```python
from build123d import *

# Parameters (mm, degrees)
F1_DEPTH = 24
F2_R     = 1.98374
F3_R     = 3.69316
F4_R     = 3.96875
F5_R     = 0.762
F6_R     = 1.8288
F7_DEPTH = 1.70942


with BuildPart() as f1:
    # F0 (on Top) → F1 (new body)
    with BuildSketch(Plane.XY):
        Polygon((0, -13.29058), (0, 0), (9.92124, 0), (9.92124, 1.70942), (-1.70942, 1.70942), (-1.70942, -11.58116), (-16.70942, -11.58116), (-16.70942, -13.29058), align=None)
    extrude(amount=F1_DEPTH)

    # F2
    f2_edges = [f1.edges().sort_by_distance(p)[0] for p in [
        (0, 0, 12),
        (-1.70942, -11.58116, 12),
    ]]
    fillet(f2_edges, radius=F2_R)

    # F3
    f3_edges = [f1.edges().sort_by_distance(p)[0] for p in [
        (0, -13.29058, 12),
        (-1.70942, 1.70942, 12),
    ]]
    fillet(f3_edges, radius=F3_R)

    # F4
    f4_edges = [f1.edges().sort_by_distance(p)[0] for p in [
        (9.92124, 0.85471, 24),
        (9.92124, 0.85471, 0),
    ]]
    fillet(f4_edges, radius=F4_R)

    # F5
    f5_edges = [f1.edges().sort_by_distance(p)[0] for p in [
        (-16.70942, -12.43587, 0),
        (-16.70942, -12.43587, 24),
    ]]
    fillet(f5_edges, radius=F5_R)

    # F6 (on face) → F7 (cut, through all)
    with BuildSketch(Plane.XZ):
        with Locations((5.95249, 20.03125)):
            Circle(F6_R)
        with Locations((5.95249, 3.96875)):
            Circle(F6_R)
    extrude(amount=-F7_DEPTH, mode=Mode.SUBTRACT)


solid = f1.part
```
The model under review builds one solid part; all positions refer to its coordinate system, in mm. A direction names the side the tool comes from. Give positions to 0.01 mm unless a question says otherwise; leave off trailing zeros. Write each loop counter-clockwise with the first axis right and the second up, starting at its lowest first coordinate (ties: lowest second). Pieces come first, ordered by that corner, then holes. Notation, with made-up numbers: (-27.75, 59) - (26.25, 59) arc R21 ccw to (26.25, 85) - close; hole circle Ø6 at (37.25, 22). An arc over 180 degrees is marked (long way). Answer in a Markdown table with one row per item. Add a question column.
1. We need section D-D on y = -8.25. Write out the cut boundary in (x, z), then the cut area to 3 significant figures.
2. Wall thickness on line 1 along Y through (x, z) = (7.5, 1.75); line 2 along Y through (x, z) = (-8.5, 2); line 3 along X through (y, z) = (-6.75, 22): over which ranges is each line inside the solid? List them lowest first. Write a range as [from, to].
3. Insertion check: P1, Ø4, axis at y = -7, z = 18, coming from the +X side; P2, Ø6.5, axis at x = -8.5, z = 12.5, coming from the +Y side; P3, Ø1.5, axis at y = -10, z = 17, coming from the -X side. Each pin has a flat end and moves straight along its axis. Give the tip position at first contact, or say it passes through.
4. Tool access review of faces 1 (the flat face through (-1.709, -6, 12)), 2 (the flat face through (0, -6, 12)), 3 (the flat face through (-10, -13.291, 12)): name each direction out of +Z, -Z, +X, -X, +Y, -Y from which nothing blocks a thin tool from reaching the whole face with its end or side.
5. We need section A-A on z = 6.75. Write out the cut boundary in (x, y).
6. We need section B-B on x = 5.5. Write out the cut boundary in (y, z), then the cut area to 3 significant figures.
7. Draft analysis for pull direction X (two halves, no side actions). For faces 4 (the cylindrical face through (5.714, 0.843, 21.844)), 5 (the flat face through (-16.709, -12, 12)), 6 (the flat face through (9.921, 1, 12)), state which applies: +X half, -X half, draft (parallel to the pull), parting line (faces both ways), or undercut.
8. We need section C-C on z = 3. Write out the cut boundary in (x, y).
Ans:
| question | item | result |
|---|---|---|
| 1 | outline | (-1.71, 0) - (0, 0) - (0, 24) - (-1.71, 24) - close |
| 1 | area | 41.0 mm^2 |
| 2 | line 1 | y = [0, 1.71] |
| 2 | line 2 | y = [-13.29, -11.58] |
| 2 | line 3 | x = [-1.71, 0] |
| 3 | P1 | stops at x = 0 |
| 3 | P2 | stops at y = -11.58 |
| 3 | P3 | stops at x = -2.08 |
| 4 | face 1 | +Z, -Z, -X, +Y |
| 4 | face 2 | +Z, -Z, +X, -Y |
| 4 | face 3 | +Z, -Z, +X, -X, -Y |
| 5 | outline | (-16.71, -13.29) - (-3.69, -13.29) arc R3.69 ccw to (0, -9.6) - (0, -1.98) arc R1.98 cw to (1.98, 0) - (9.92, 0) - (9.92, 1.71) - (1.98, 1.71) arc R3.69 ccw to (-1.71, -1.98) - (-1.71, -9.6) arc R1.98 cw to (-3.69, -11.58) - (-16.71, -11.58) - close |
| 6 | outline | (0, 0) - (1.71, 0) - (1.71, 2.2) - (0, 2.2) - close; (0, 5.74) - (1.71, 5.74) - (1.71, 18.26) - (0, 18.26) - close; (0, 21.8) - (1.71, 21.8) - (1.71, 24) - (0, 24) - close |
| 6 | area | 28.9 mm^2 |
| 7 | face 4 | undercut |
| 7 | face 5 | -X half |
| 7 | face 6 | +X half |
| 8 | outline | (-16.71, -13.29) - (-3.69, -13.29) arc R3.69 ccw to (0, -9.6) - (0, -1.98) arc R1.98 cw to (1.98, 0) - (4.4, 0) - (4.4, 1.71) - (1.98, 1.71) arc R3.69 ccw to (-1.71, -1.98) - (-1.71, -9.6) arc R1.98 cw to (-3.69, -11.58) - (-16.71, -11.58) - close; (7.5, 0) - (9.8, 0) - (9.8, 1.71) - (7.5, 1.71) - close |
